Could you check a few things on this drawing? It's one solid part, dimensions in mm from its lowest x, y, z. Round coordinates to 2 decimals unless told otherwise and drop trailing zeros. Write each loop counter-clockwise with the first axis right and the second up, starting at its lowest first coordinate (ties: lowest second). Pieces come first, ordered by that corner, then holes. Notation, with made-up numbers: (-10, 74.25) -> (14, 74.25) arc R31 ccw to (14, 100.25) -> close; hole circle Ø7 at (-36, -10.75). An arc over 180 degrees is marked (long way). Answer in a Markdown table with one row per item.
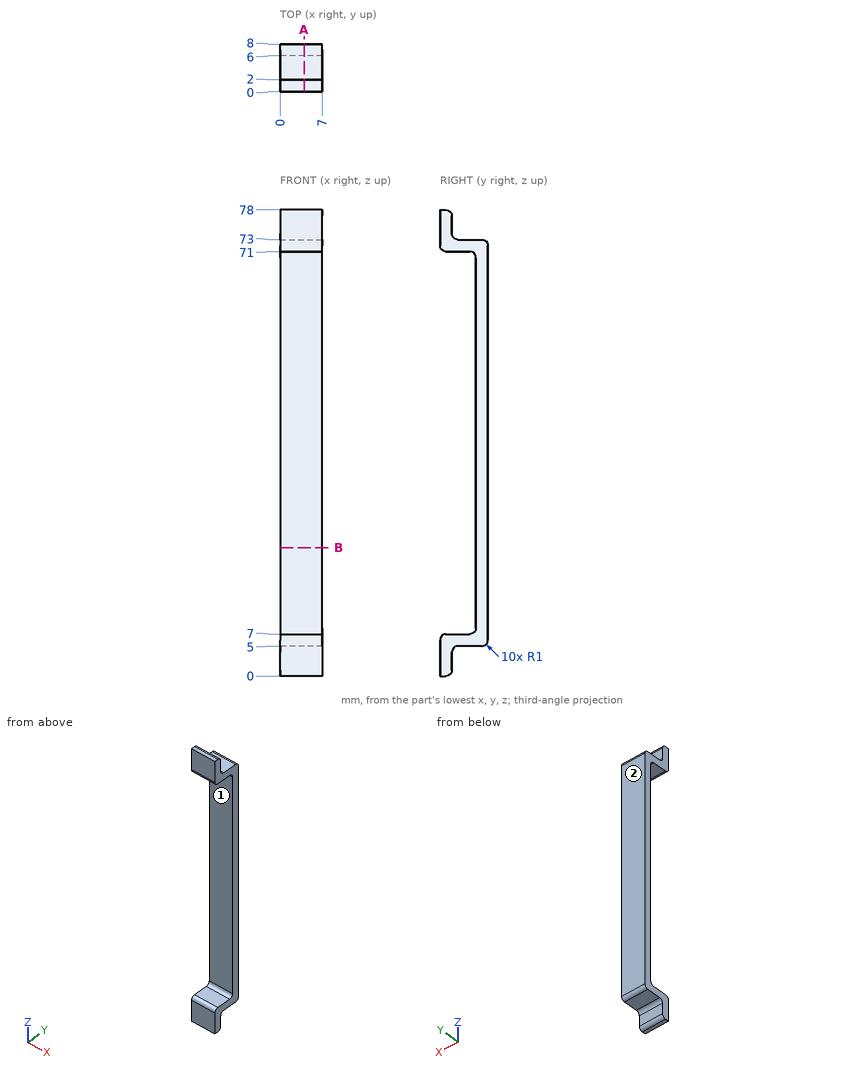
1) I need wall thicknesses on line 1 (Z direction, x = 6.25, y = 4.5); line 2 (Z direction, x = 5.75, y = 5.5); line 3 (Y direction, x = 2.5, z = 14). Which ranges of each line are inside material? Lowest first, please. Write a range as [from, to].
Response:
| item | result |
|---|---|
| line 1 | z = [5, 7], [71, 73] |
| line 2 | z = [5, 7.13], [70.87, 73] |
| line 3 | y = [6, 8] |
2) I want a section at A-A, the plane x = 4. List the corners of the cut face in (y, z) for me, and give its area (3 significant figures).
Response:
| item | result |
|---|---|
| outline | (0, 0) -> (1, 0) arc R1 ccw to (2, 1) -> (2, 4) arc R1 cw to (3, 5) -> (7, 5) arc R1 ccw to (8, 6) -> (8, 72) arc R1 ccw to (7, 73) -> (3, 73) arc R1 cw to (2, 74) -> (2, 77) arc R1 ccw to (1, 78) -> (0, 78) -> (0, 72) arc R1 ccw to (1, 71) -> (5, 71) arc R1 cw to (6, 70) -> (6, 8) arc R1 cw to (5, 7) -> (1, 7) arc R1 ccw to (0, 6) -> close |
| area | 180 mm^2 |
3) I want a section at B-B, the plane z = 21.5. List the corners of the cut face in (x, y) for me, and give its area (3 significant figures).
Response:
| item | result |
|---|---|
| outline | (0, 6) -> (7, 6) -> (7, 8) -> (0, 8) -> close |
| area | 14.0 mm^2 |
4) We'd pull the mould along Z, two halves only. Please class the marked faces 1 and 2: +Z half, -Z half, draft (parallel to the pull), parting line (faces both ways), or undercut.
Response:
| item | result |
|---|---|
| face 1 | undercut |
| face 2 | draft |
5) For pin 1 (1.5 mm diameter, centred on x = 3.5, y = 5.5, fed in from +Z); pin 2 (2.5 mm diameter, centred on x = 4.5, z = 3, fed in from +Y); pin 3 (3 mm diameter, centred on x = 2.5, z = 27, fed in from -Y); pin 4 (2 mm diameter, centred on y = 4, z = 68.5, fed in from +X), each with a flat end and sliding along its axis, tell me the tip position at first contact or that it passes through.
Response:
| item | result |
|---|---|
| pin 1 | stops at z = 73 |
| pin 2 | stops at y = 2.03 |
| pin 3 | stops at y = 6 |
| pin 4 | passes through |
